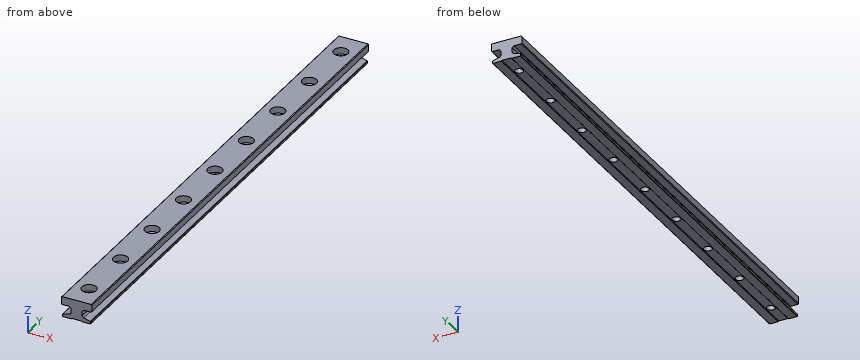
from build123d import *

# Parameters (mm, degrees)
AUFSATZ_LINEAR_AUSTRAGEN1_DEPTH                     = 220
STIRNSENKUNG_F_R_M3_SECHSKANTSCHRAUBE_G_D           = 3.4
STIRNSENKUNG_F_R_M3_SECHSKANTSCHRAUBE_G_CBORE_D     = 6.1
STIRNSENKUNG_F_R_M3_SECHSKANTSCHRAUBE_G_CBORE_DEPTH = 2.7
FORMSCHR_GE1_ANGLE                                  = 45


with BuildPart() as part:
    # Skizze1 → Aufsatz-Linear austragen1 (new body)
    with BuildSketch(Plane(origin=(0, 25, 0), x_dir=(1, 0, 0), z_dir=(0, 1, 0))):
        with BuildLine():
            Line((1.959999996, -0.240000001), (-1.960000004, -0.240000001))
            Line((-1.960000004, -0.240000001), (-1.960000004, -1e-09))
            Line((-1.960000004, -1e-09), (-5.840000004, -1e-09))
            ThreePointArc((-5.840000004, -1e-09), (-5.953137089, -0.046862916), (-6.000000004, -0.160000001))
            Line((-6.000000004, -0.160000001), (-6.000000004, -0.946534601))
            ThreePointArc((-6.000000004, -0.946534601), (-5.958670671, -1.068286889), (-5.85176381, -1.13971977))
            Line((-5.85176381, -1.13971977), (-2.992944765, -1.905738019))
            ThreePointArc((-2.992944765, -1.905738019), (-2.565317328, -2.191469536), (-2.4, -2.67847868))
            Line((-2.4, -2.67847868), (-2.4, -4.5))
            Line((-2.4, -4.5), (-3.1, -5.2))
            Line((-3.1, -5.2), (-6.2, -5.2))
            Line((-6.2, -5.2), (-6.5, -5.5))
            Line((-6.5, -5.5), (-6.5, -8.28))
            Line((-6.5, -8.28), (-6.18, -8.6))
            Line((-6.18, -8.6), (6.18, -8.6))
            Line((6.18, -8.6), (6.5, -8.28))
            Line((6.5, -8.28), (6.5, -5.5))
            Line((6.5, -5.5), (6.2, -5.2))
            Line((6.2, -5.2), (3.1, -5.2))
            Line((3.1, -5.2), (2.4, -4.5))
            Line((2.4, -4.5), (2.4, -2.67847868))
            ThreePointArc((2.4, -2.67847868), (2.565317328, -2.191469536), (2.992944765, -1.905738019))
            Line((2.992944765, -1.905738019), (5.851763809, -1.139719768))
            ThreePointArc((5.851763809, -1.139719768), (5.958670669, -1.068286888), (6.000000002, -0.946534601))
            Line((6.000000002, -0.946534601), (6.000000002, -0.160000001))
            ThreePointArc((6.000000002, -0.160000001), (5.953137087, -0.046862916), (5.840000002, -1e-09))
            Line((5.840000002, -1e-09), (1.959999996, -1e-09))
            Line((1.959999996, -1e-09), (1.959999996, -0.240000001))
        make_face()
    extrude(amount=-AUFSATZ_LINEAR_AUSTRAGEN1_DEPTH)

    # Stirnsenkung für M3 Sechskantschraube, Gewinde bis Kopf1 (through all)
    with Locations(Plane.XY.offset(8.6)):
        with Locations((0, -85), (0, -60), (0, -35), (0, -10), (0, 15), (0, -110), (0, -135), (0, -160), (0, -185)):
            CounterBoreHole(STIRNSENKUNG_F_R_M3_SECHSKANTSCHRAUBE_G_D / 2, STIRNSENKUNG_F_R_M3_SECHSKANTSCHRAUBE_G_CBORE_D / 2, STIRNSENKUNG_F_R_M3_SECHSKANTSCHRAUBE_G_CBORE_DEPTH)

    # Formschräge1
    formschr_ge1_faces = [part.faces().sort_by_distance(p)[0] for p in [
        (-1.960000004, -85, 0.120000001),
        (1.959999996, -85, 0.120000001),
    ]]
    draft(formschr_ge1_faces, Plane(origin=(1.959999996, -195, 0.240000001), x_dir=(-1, 0, 0), z_dir=(0, 0, -1)), FORMSCHR_GE1_ANGLE)


solid = part.part
Geometry check sheet. Reference: the model listing, model coordinates, mm. Round coordinates to 2 decimals unless told otherwise and drop trailing zeros. Order: outer loops, then holes, each group sorted by start corner. A loop starts at its lowest first (then second) coordinate and runs counter-clockwise, first axis right, second up. Notation, with made-up numbers: M -30.5,9 L -7.5,9 A19 ccw -7.5,16 Z; hole C 77,36.5 d10. An arc over 180 degrees is marked long. Answer in a Markdown table with one row per item. Add a question column.
Item 1: Depth check by flat-ended pin: pin 1 Ø4.5 at (x, y) = (0, -135) entering from +Z; pin 2 Ø4 at (x, y) = (0, -85) entering from -Z; pin 3 Ø2.5 at (x, y) = (0, 15) entering from -Z; pin 4 Ø1.5 at (y, z) = (0, 3) entering from +X. Enter the tip coordinate at first touch or a pass-through.
Item 2: Material ranges on L1, parallel to X at y = -185, z = 3.15; L2, parallel to X at y = -133, z = 4.5; L3, parallel to Z at x = -1.75, y = 12, recorded low to high. Write a range as [from, to].
Item 3: Sectioned sample at A-A, the plane y = -0.5. Enter the section's corners in (x, z), plus the area to 3 significant figures.
Filled in:
| question | item | result |
|---|---|---|
| 1 | pin 1 | stops at z = 5.9 |
| 1 | pin 2 | stops at z = 0.2 |
| 1 | pin 3 | passes through |
| 1 | pin 4 | stops at x = 2.52 |
| 2 | L1 | x = [-2.4, -1.7], [1.7, 2.4] |
| 2 | L2 | x = [-2.4, 2.4] |
| 2 | L3 | z = [0.24, 8.6] |
| 3 | outline | M -6.5,5.5 L -6.2,5.2 L -3.1,5.2 L -2.4,4.5 L -2.4,2.68 A0.8 cw -2.99,1.91 L -5.85,1.14 A0.2 ccw -6,0.95 L -6,0.16 A0.16 ccw -5.84,0 L -2.2,0 L -1.96,0.24 L 1.96,0.24 L 2.2,0 L 5.84,0 A0.16 ccw 6,0.16 L 6,0.95 A0.2 ccw 5.85,1.14 L 2.99,1.91 A0.8 cw 2.4,2.68 L 2.4,4.5 L 3.1,5.2 L 6.2,5.2 L 6.5,5.5 L 6.5,8.28 L 6.18,8.6 L -6.18,8.6 L -6.5,8.28 Z |
| 3 | area | 80.0 mm² |
